```python
from build123d import *

# Parameters (mm, degrees)
SKETCH1_R           = 23
BOSS_EXTRUDE1_DEPTH = 120
SKETCH2_R           = 14.5
CUT_EXTRUDE1_DEPTH  = 120
CUT_EXTRUDE2_DEPTH  = 2.5
SKETCH5_R           = 1.75
CUT_EXTRUDE3_DEPTH  = 10
BOSS_EXTRUDE2_START = -5
SKETCH6_R           = 14.5
BOSS_EXTRUDE2_DEPTH = 5
SKETCH7_R           = 4
CUT_EXTRUDE4_DEPTH  = 5


with BuildPart() as part:
    # Sketch1 → Boss-Extrude1 (new body)
    with BuildSketch(Plane(origin=(0, 0, 0), x_dir=(1, 0, 0), z_dir=(0, 1, 0))):
        with Locations(Location((0, 0, 0), (0, 0, 270))):
            Circle(SKETCH1_R)
    extrude(amount=BOSS_EXTRUDE1_DEPTH)

    # Sketch2 → Cut-Extrude1 (cut)
    with BuildSketch(Plane(origin=(0, 120, 0), x_dir=(1, 0, 0), z_dir=(0, 1, 0))):
        with Locations(Location((0, 0, 0), (0, 0, 270))):
            Circle(SKETCH2_R)
    extrude(amount=-CUT_EXTRUDE1_DEPTH, mode=Mode.SUBTRACT)

    # Sketch4 → Cut-Extrude2 (cut)
    with BuildSketch(Plane(origin=(0, 120, 0), x_dir=(1, 0, 0), z_dir=(0, 1, 0))):
        Polygon((-14, 0), (-15.75, -3.031088913), (-19.25, -3.031088913), (-21, 0), (-19.25, 3.031088913), (-15.75, 3.031088913), align=None)
        Polygon((19.25, 3.031088913), (15.75, 3.031088913), (14, 0), (15.75, -3.031088913), (19.25, -3.031088913), (21, 0), align=None)
    extrude(amount=-CUT_EXTRUDE2_DEPTH, mode=Mode.SUBTRACT)

    # Sketch5 → Cut-Extrude3 (cut)
    with BuildSketch(Plane(origin=(0, 117.5, 0), x_dir=(1, 0, 0), z_dir=(0, 1, 0))):
        with Locations(Location((-17.5, 0, 0), (0, 0, 270))):
            Circle(SKETCH5_R)
        with Locations(Location((17.5, 0, 0), (0, 0, 90))):
            Circle(SKETCH5_R)
    extrude(amount=-CUT_EXTRUDE3_DEPTH, mode=Mode.SUBTRACT)

    # Sketch6 → Boss-Extrude2 (add)
    with BuildSketch(Plane(origin=(0, 0, 0), x_dir=(-1, 0, 0), z_dir=(0, -1, 0)).offset(BOSS_EXTRUDE2_START)):
        with Locations(Location((0, 0, 0), (0, 0, 183.262923921))):
            Circle(SKETCH6_R)
    extrude(amount=BOSS_EXTRUDE2_DEPTH)

    # Sketch7 → Cut-Extrude4 (cut)
    with BuildSketch(Plane.XZ):
        with Locations(Location((0, 0, 0), (0, 0, 270))):
            Circle(SKETCH7_R)
    extrude(amount=-CUT_EXTRUDE4_DEPTH, mode=Mode.SUBTRACT)


solid = part.part
```
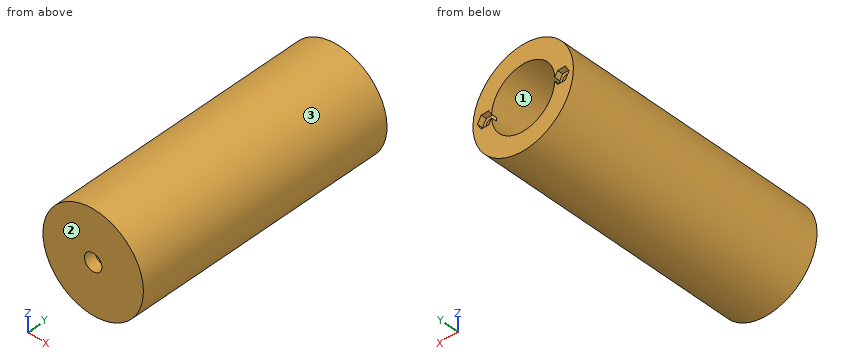
Geometry: final body of the model. Coordinates: model frame, mm. Face numbers are marked on the shaded views. Round coordinates to 2 decimals unless told otherwise and drop trailing zeros. Loops run counter-clockwise (first coordinate to the right, second up) from the corner with the lowest first, then second, coordinate; pieces in that order, holes last.
Item 1: Contact query for flat-ended pins moving along their axis: P1, Ø1.2, axis at x = -17.5, y = 119, coming from the -Z side; P2, Ø1.8, axis at x = -17, z = 0.5, coming from the +Y side; P3, Ø13, axis at x = 0, z = 0, coming from the +Y side. Output: stop coordinate, or through.
Checked values:
P1: stops at z = -15.6
P2: stops at y = 107.5
P3: stops at y = 5
Item 2: Mould query, pull axis Z, two halves, no side actions, for the marked faces 1, 2 and 3. Classes: released by +Z, released by -Z, zero draft, split by the parting line, or undercut.
Checked values:
face 1: undercut
face 2: zero draft
face 3: split by the parting line
Item 3: Section C-C, the plane z = 9. Output: boundary loops of the cut face in (x, y), plus the area to 3 significant figures.
Checked values:
outline: (-21.17, 0) - (21.17, 0) - (21.17, 120) - (11.37, 120) - (11.37, 5) - (-11.37, 5) - (-11.37, 120) - (-21.17, 120) - close
area: 2,470 mm2
Item 4: Section A-A, the plane x = 0. Output: boundary loops of the cut face in (y, z), plus the area to 4 significant figures.
Checked values:
outline: (0, -23) - (120, -23) - (120, -14.5) - (5, -14.5) - (5, -4) - (0, -4) - close; (0, 4) - (5, 4) - (5, 14.5) - (120, 14.5) - (120, 23) - (0, 23) - close
area: 2,145 mm2
Item 5: Section B-B, the plane y = 74. Output: boundary loops of the cut face in (x, z), plus the area to 3 significant figures.
Checked values:
outline: circle Ø46 at (0, 0); hole circle Ø29 at (0, 0)
area: 1,000 mm2
Item 6: Line query: L1, parallel to X at y = 114.5, z = 0; L2, parallel to X at y = 51.5, z = -1; L3, parallel to X at y = 30, z = 5. Output: solid intervals per line, ascending.
Checked values:
L1: x = -23 to -19.25, -15.75 to -14.5, 14.5 to 15.75, 19.25 to 23
L2: x = -22.98 to -14.47, 14.47 to 22.98
L3: x = -22.45 to -13.61, 13.61 to 22.45
Item 7: Section D-D, the plane x = 17.5. Output: boundary loops of the cut face in (y, z), plus the area to 3 significant figures.
Checked values:
outline: (0, -14.92) - (120, -14.92) - (120, -3.03) - (117.5, -3.03) - (117.5, -1.75) - (107.5, -1.75) - (107.5, 1.75) - (117.5, 1.75) - (117.5, 3.03) - (120, 3.03) - (120, 14.92) - (0, 14.92) - close
area: 3,530 mm2
